The listing builds one solid part. Answer for the finished solid, in the listing's coordinates (mm). A direction names the side the tool comes from. Coordinates: 2 decimals unless noted, no trailing zeros. Loops run counter-clockwise (first coordinate to the right, second up) from the corner with the lowest first, then second, coordinate; pieces in that order, holes last. Notation, with made-up numbers: (41.5, 46) - (71.5, 46) arc R22 cw to (71.5, 59) - close; hole circle Ø6 at (75, 71). An arc over 180 degrees is marked (long way). One line per question, with ' | ' between items.
from build123d import *

# Parameters (mm, degrees)
BOSS_EXTRUDE1_DEPTH = 558.8
CUT_EXTRUDE1_REACH  = 561.953
SKETCH2_R           = 7.9375
CUT_EXTRUDE2_REACH  = 561.953
SKETCH3_R           = 7.9375


with BuildPart() as part:
    # Sketch1 → Boss-Extrude1 (new body)
    with BuildSketch(Plane.XY):
        Polygon((-22.225, -9.525), (-22.225, 12.7), (-25.4, 12.7), (-25.4, -12.7), (25.4, -12.7), (25.4, 12.7), (22.225, 12.7), (22.225, -9.525), align=None)
    extrude(amount=BOSS_EXTRUDE1_DEPTH)

    # Sketch2 → Cut-Extrude1 (cut, up to next)
    with BuildSketch(Plane.XZ.offset(12.7), mode=Mode.PRIVATE) as cut_extrude1_sk1:
        with Locations((0, 33.3375)):
            Circle(SKETCH2_R)
    cut_extrude1_tool1 = extrude(cut_extrude1_sk1.sketch, amount=-CUT_EXTRUDE1_REACH, mode=Mode.PRIVATE) & part.part
    add(cut_extrude1_tool1.solids().sort_by_distance((0, -12.7, 33.3375))[0], mode=Mode.SUBTRACT)

    # Sketch3 → Cut-Extrude2 (cut, up to next)
    with BuildSketch(Plane.XZ.offset(12.7), mode=Mode.PRIVATE) as cut_extrude2_sk1:
        with Locations((0, 538.1625)):
            Circle(SKETCH3_R)
    cut_extrude2_tool1 = extrude(cut_extrude2_sk1.sketch, amount=-CUT_EXTRUDE2_REACH, mode=Mode.PRIVATE) & part.part
    add(cut_extrude2_tool1.solids().sort_by_distance((0, -12.7, 538.1625))[0], mode=Mode.SUBTRACT)


solid = part.part
Item 1: Each of these flat-tipped pins is pushed along its axis until it touches: pin 1 Ø18.5 at (x, z) = (0, 538.16) entering from +Y (3 decimals); pin 2 Ø12.5 at (x, z) = (0, 33.34) entering from -Y. Where does it stop, or does it pass through?
Taken from the geometry:
pin 1: stops at y = -9.525 | pin 2: passes through
Item 2: Find section B-B, the plane y = 5. Write down the section's boundary in (x, z) (3 decimals), plus the area to 3 significant figures.
Taken from the geometry:
outline: (-25.4, 0) - (-22.225, 0) - (-22.225, 558.8) - (-25.4, 558.8) - close; (22.225, 0) - (25.4, 0) - (25.4, 558.8) - (22.225, 558.8) - close | area: 3,550 mm2
Item 3: Find section A-A, the plane x = 0. Write down the section's boundary in (y, z) (3 decimals), plus the area to 3 significant figures.
Taken from the geometry:
outline: (-12.7, 0) - (-9.525, 0) - (-9.525, 25.4) - (-12.7, 25.4) - close; (-12.7, 41.275) - (-9.525, 41.275) - (-9.525, 530.225) - (-12.7, 530.225) - close; (-12.7, 546.1) - (-9.525, 546.1) - (-9.525, 558.8) - (-12.7, 558.8) - close | area: 1,670 mm2
Item 4: Find section C-C, the plane z = 469. Write down the section's boundary in (x, y) (3 decimals).
Taken from the geometry:
outline: (-25.4, -12.7) - (25.4, -12.7) - (25.4, 12.7) - (22.225, 12.7) - (22.225, -9.525) - (-22.225, -9.525) - (-22.225, 12.7) - (-25.4, 12.7) - close
Item 5: The mould has two halves that part along Z. Classify faces 1 (the face through (-1.033, -11.135, 41.207)), 2 (the face through (25.4, 0, 275)), 3 (the face through (2, -10, 0)): pulls with the +Z half, pulls with the -Z half, needs draft (parallel to the pull), parting line crosses it, or undercut.
Taken from the geometry:
face 1: undercut | face 2: needs draft | face 3: pulls with the -Z half
Item 6: Which of the six approach directions +Z, -Z, +X, -X, +Y, -Y give full straight-line access (tool end or side, diameter ignored) to faces 4 (the face through (-1.033, -11.135, 546.032)), 5 (the face through (-22.225, 1, 275))?
Taken from the geometry:
face 4: +Y, -Y | face 5: +Z, -Z, +Y
Item 7: Find the intervals of material crossed by line 1 (Z direction, x = 0, y = -10.5) (3 decimals); line 2 (X direction, y = 7.5, z = 119.5) (3 decimals); line 3 (Y direction, x = -3.5, z = 89.5) (3 decimals), in increasing order. Write a range as [from, to].
Taken from the geometry:
line 1: z = [0, 25.4], [41.275, 530.225], [546.1, 558.8] | line 2: x = [-25.4, -22.225], [22.225, 25.4] | line 3: y = [-12.7, -9.525]
